```python
from build123d import *

# Parameters (mm, degrees)
BOSS_EXTRUDE1_DEPTH = 300
SKETCH2_R           = 2.25
CUT_EXTRUDE1_DEPTH  = 10
SKETCH3_R           = 2.25
CUT_EXTRUDE2_DEPTH  = 10


with BuildPart() as part:
    # Sketch1 → Boss-Extrude1 (new body)
    with BuildSketch(Plane(origin=(0, 0, 0), x_dir=(1, 0, 0), z_dir=(0, 1, 0))):
        Polygon((-12.7, 0), (0, 0), (0, 12.7), (-3.18, 12.7), (-3.18, 3.18), (-12.7, 3.18), align=None)
    extrude(amount=BOSS_EXTRUDE1_DEPTH)

    # Sketch2 → Cut-Extrude1 (cut)
    with BuildSketch(Plane.ZY.offset(3.18)):
        with Locations((-7.94, 275)):
            Circle(SKETCH2_R)
        with Locations((-7.94, 175)):
            Circle(SKETCH2_R)
        with Locations((-7.94, 75)):
            Circle(SKETCH2_R)
    extrude(amount=-CUT_EXTRUDE1_DEPTH, mode=Mode.SUBTRACT)

    # Sketch3 → Cut-Extrude2 (cut)
    with BuildSketch(Plane(origin=(0, 0, -3.18), x_dir=(-1, 0, 0), z_dir=(0, 0, -1))):
        with Locations((7.94, 225)):
            Circle(SKETCH3_R)
        with Locations((7.94, 125)):
            Circle(SKETCH3_R)
        with Locations((7.94, 25)):
            Circle(SKETCH3_R)
    extrude(amount=-CUT_EXTRUDE2_DEPTH, mode=Mode.SUBTRACT)


solid = part.part
```
CAD build for the part. Positions are in the model's coordinates, mm. A direction names the side the tool comes from. Coordinates: 2 decimals unless noted, no trailing zeros. Write each loop counter-clockwise with the first axis right and the second up, starting at its lowest first coordinate (ties: lowest second). Pieces come first, ordered by that corner, then holes. Notation, with made-up numbers: (17.25, 19.25) -> (48.25, 19.25) arc R29 ccw to (48.25, 51.25) -> close; hole circle Ø6 at (5.25, 35). An arc over 180 degrees is marked (long way). Use CSV: the item, a comma, the result in double quotes. Start each with the question number.
Item 1: Tool access for faces 1 (the flat face through (-4, 300, -2)), 2 (the flat face through (-8, 148, -3.18)): list every direction of +Z, -Z, +X, -X, +Y, -Y with a clear straight run to the whole face (end or side of a thin tool).
Item 2: Band-saw the part on A-A, the plane z = -7.94. Write the cut outline in (x, y), plus the area to 3 significant figures.
Item 3: Band-saw the part on B-B, the plane y = 98. Write the cut outline in (x, z).
Item 4: Drop flat-ended pins along their axis: P1, Ø1.5, axis at x = -2.5, y = 53.5, coming from the +Z side; P2, Ø3, axis at x = -9.5, y = 131.5, coming from the -Z side; P3, Ø5, axis at y = 215, z = -6.5, coming from the -X side. Give the stop position or say it passes through.
Item 5: Wall check: probe 1 along Y at (x, z) = (-7.94, -1.4); probe 2 along Y at (x, z) = (-0.7, -7.94); probe 3 along Z at (x, y) = (-2.1, 175). Give the ranges that are in metal, low to high.
Response values:
1,face 1,"+Z, -Z, +X, -X, +Y"
1,face 2,"-Z, -X, +Y, -Y"
2,outline,"(-3.18, 0) -> (0, 0) -> (0, 72.75) -> (-3.18, 72.75) -> close; (-3.18, 77.25) -> (0, 77.25) -> (0, 172.75) -> (-3.18, 172.75) -> close; (-3.18, 177.25) -> (0, 177.25) -> (0, 272.75) -> (-3.18, 272.75) -> close; (-3.18, 277.25) -> (0, 277.25) -> (0, 300) -> (-3.18, 300) -> close"
2,area,"911 mm2"
3,outline,"(-12.7, -3.18) -> (-3.18, -3.18) -> (-3.18, -12.7) -> (0, -12.7) -> (0, 0) -> (-12.7, 0) -> close"
4,P1,"stops at z = 0"
4,P2,"stops at z = -3.18"
4,P3,"stops at x = -3.18"
5,probe 1,"y = 0 to 22.75, 27.25 to 122.75, 127.25 to 222.75, 227.25 to 300"
5,probe 2,"y = 0 to 72.75, 77.25 to 172.75, 177.25 to 272.75, 277.25 to 300"
5,probe 3,"z = -12.7 to -10.19, -5.69 to 0"
